Geometry check sheet. Reference: the model listing, model coordinates, mm. Give positions to 0.01 mm unless a question says otherwise; leave off trailing zeros. Loops run counter-clockwise (first coordinate to the right, second up) from the corner with the lowest first, then second, coordinate; pieces in that order, holes last. Notation, with made-up numbers: (55.5, 80.25) - (76.5, 80.25) arc R10 ccw to (76.5, 93.25) - close; hole circle Ø8 at (33, 76.25). An arc over 180 degrees is marked (long way). Use a Markdown table: item, result. Add a question column.
1. Material ranges on L1, parallel to Y at x = 0, z = 12.7; L2, parallel to Y at x = 0.5, z = 14.5; L3, parallel to X at y = 17.5, z = 21.5, recorded low to high.
2. Cross-section at C-C on z = 16.75. Enter the section's corners in (x, y), and give its area (3 significant figures).
3. Depth check by flat-ended pin: P1, Ø1, axis at x = 50, z = 7.5, coming from the +Y side; P2, Ø3, axis at x = -21, z = 17, coming from the +Y side; P3, Ø3, axis at x = -55.5, y = 44, coming from the +Z side. Enter the tip coordinate at first touch or a pass-through.
from build123d import *

# Parameters (mm, degrees)
F0_R     = 76.8798317076
F0_R_2   = 21.949412209
F1_DEPTH = 25.4
F2_R     = 12.7
F3_R     = 12.69999
F4_R     = 12.7
F5_R     = 12.69999


# Not quite as in the source:
# - a fillet or chamfer is up to 0.001 mm smaller than in the source, because OpenCascade refuses the exact size


with BuildPart() as f1:
    # F0 (on Top) → F1 (new body)
    with BuildSketch(Plane.XY):
        Circle(F0_R)
        Circle(F0_R_2, mode=Mode.SUBTRACT)
    extrude(amount=F1_DEPTH)

    # F2
    f2_edges = [f1.edges().sort_by_distance(p)[0] for p in [
        (-76.879832, 0, 25.4),
    ]]
    fillet(f2_edges, radius=F2_R)

    # F3 (radius 12.7 in the source; OpenCascade refuses exactly that, so slightly less here)
    f3_edges = [f1.edges().sort_by_distance(p)[0] for p in [
        (-76.879832, 0, 0),
    ]]
    fillet(f3_edges, radius=F3_R)

    # F4
    f4_edges = [f1.edges().sort_by_distance(p)[0] for p in [
        (-21.949412, 0, 25.4),
    ]]
    fillet(f4_edges, radius=F4_R)

    # F5 (radius 12.7 in the source; OpenCascade refuses exactly that, so slightly less here)
    f5_edges = [f1.edges().sort_by_distance(p)[0] for p in [
        (-21.949412, 0, 0),
    ]]
    fillet(f5_edges, radius=F5_R)


solid = f1.part
Values found:
| question | item | result |
|---|---|---|
| 1 | L1 | y = -76.88 to -21.95, 21.95 to 76.88 |
| 1 | L2 | y = -76.75 to -22.07, 22.07 to 76.75 |
| 1 | L3 | x = -71.22 to -18.54, 18.54 to 71.22 |
| 2 | outline | circle Ø152.43 at (0, 0); hole circle Ø45.22 at (0, 0) |
| 2 | area | 16,600 mm2 |
| 3 | P1 | stops at y = 57.45 |
| 3 | P2 | stops at y = 73.81 |
| 3 | P3 | stops at z = 24.31 |
